```python
from build123d import *

# Parameters (mm, degrees)
F0_W        = 65.5969455838
F0_H        = 62.3628050089
F1_DEPTH    = 50.8
F3_DEPTH    = 101.6
F4_W        = 40.8792179078
F4_H        = 14.0294057783
F5_DEPTH    = 2.54
F6_R        = 5.8595306003
F7_DEPTH    = 25.4
F8_T1_DEPTH = 51.8777405358
F8_T3_DEPTH = 14.0294057783
F8_T5_DEPTH = 14.0294057783


# Not quite as in the source:
# - a fillet or chamfer that OpenCascade refuses, or shapes differently, is made with other operations: its cross-section is extruded or revolved along the edge and cut away or added


with BuildPart() as f1:
    # F0 (on Top) → F1 (new body)
    with BuildSketch(Plane.XY):
        with Locations((32.7984727919, 31.1814025044)):
            Rectangle(F0_W, F0_H)
    extrude(amount=F1_DEPTH)

    # F2 (on face) → F3 (cut)
    with BuildSketch(Plane.XZ):
        Polygon((89.7827520967, 45.4889908433), (33.5367023945, 62.9252642393), (74.5963230729, 21.5844195336), align=None)
    extrude(amount=-F3_DEPTH, mode=Mode.SUBTRACT)

    # F4 (on face) → F5 (cut)
    with BuildSketch(Plane(origin=(48.3447062482, 0, 48.0158379562), x_dir=(0, 1, 0), z_dir=(0.7095159293, 0, 0.7046893969))):
        with Locations((30.5939735845, -10.8757299604)):
            Rectangle(F4_W, F4_H)
    extrude(amount=-F5_DEPTH, mode=Mode.SUBTRACT)

    # F6 (on face) → F7 (cut)
    with BuildSketch(Plane.XZ):
        with Locations((31.5736755729, 25.0635799021)):
            Circle(F6_R)
    extrude(amount=-F7_DEPTH, mode=Mode.SUBTRACT)

    # F8: fillet of radius 5.08 on 4 edges, made by hand

    # F8_s2 → F8_t1 (join)
    with BuildSketch(Plane.XZ.offset(-62.0321051664)):
        with BuildLine():
            ThreePointArc((51.0655310864, 45.2763777457), (51.0565565883, 42.6467915619), (52.3635775369, 40.3650158763))
            Line((52.3635775369, 40.3650158763), (49.263360626, 43.4864666776))
            Line((49.263360626, 43.4864666776), (51.0655310864, 45.2763777457))
        make_face()
        with BuildLine():
            ThreePointArc((60.9519045829, 35.3222908675), (58.3223183991, 35.3312653655), (56.0495172115, 36.6538306007))
            Line((56.0495172115, 36.6538306007), (59.1497341225, 33.5323797994))
            Line((59.1497341225, 33.5323797994), (60.9519045829, 35.3222908675))
        make_face()
    extrude(amount=F8_T1_DEPTH)

    # F8_s4 → F8_t3 (join)
    with BuildSketch(Plane(origin=(12.6071983347, 0, -12.6935470887), x_dir=(0, 1, 0), z_dir=(-0.7046893969, 0, 0.7095159293))):
        with BuildLine():
            ThreePointArc((51.0335825384, -68.1375910703), (49.1741734871, -66.278182019), (46.6341734871, -65.5975910703))
            Line((46.6341734871, -65.5975910703), (51.0335825384, -65.5975910703))
            Line((51.0335825384, -65.5975910703), (51.0335825384, -68.1375910703))
        make_face()
    extrude(amount=F8_T3_DEPTH)

    # F8_s6 → F8_t5 (join)
    with BuildSketch(Plane(origin=(2.7208248382, 0, -2.7394602105), x_dir=(0, 1, 0), z_dir=(0.7046893969, 0, -0.7095159293))):
        with BuildLine():
            ThreePointArc((10.1543646306, 68.1375910703), (12.0137736818, 66.278182019), (14.5537736818, 65.5975910703))
            Line((14.5537736818, 65.5975910703), (10.1543646306, 65.5975910703))
            Line((10.1543646306, 65.5975910703), (10.1543646306, 68.1375910703))
        make_face()
    extrude(amount=F8_T5_DEPTH)


solid = f1.part
```
CAD build for the part. Positions are in the model's coordinates, mm. A direction names the side the tool comes from. Give positions to 0.01 mm unless a question says otherwise; leave off trailing zeros. Order: outer loops, then holes, each group sorted by start corner. A loop starts at its lowest first (then second) coordinate and runs counter-clockwise, first axis right, second up. Notation, with made-up numbers: M 24.5,56 L 79.5,56 A35 cw 79.5,89 Z; hole C 84.25,72.25 d5. An arc over 180 degrees is marked long. Put each result on its own line as item: value. Start each with the question number.
(1) Which spindle directions (+Z, -Z, +X, -X, +Y, -Y) get a long thin tool onto all of the face, cutting with end or side? Do faces 1 (the cylindrical face through (58.36, 30.88, 35.32)), 2 (the cylindrical face through (51.047, 30.88, 42.683)), 3 (the flat face through (32, 32, 0)). Say none if no direction does.
(2) Drill centre lines: line 1 along X through (y, z) = (5, 23); line 2 along Z through (x, y) = (46, 51); line 3 along Z through (x, y) = (48, 53). Where is each one in solid material? Low to high.
(3) Saw through at A-A, the plane z = 21.5. Write the cut outline in (x, y).
(4) Saw through at B-B, the plane y = 52.5. Write the cut outline in (x, z), then the cut area to 3 significant figures.
(5) Flat gauge pin, fed straight in: pin 1 Ø13 at (x, z) = (30, 27) entering from -Y. Where does the tip first touch, or does it go through?
(6) Saw through at D-D, the plane x = 46.5. Write the cut outline in (y, z), then the cut area to 3 significant figures.
(7) Saw through at C-C, the plane y = 4. Write the cut outline in (x, z), then the cut area to 3 significant figures.
(8) Mould opens along Y. For faces 4 (the flat face through (31, 25.4, 25)), 5 (the flat face through (54.181, 30.369, 38.535)), 6 (the cylindrical face through (54.87, 11.49, 39.3)), 7 (the cylindrical face through (36.986, 12.522, 22.819)) say: +Y half, -Y half, draft (parallel to the pull), parting line (faces both ways), or undercut.
Check result:
1. face 1: +Z
1. face 2: +X
1. face 3: -Z, +X, -X, +Y, -Y
2. line 1: x = 0 to 26.09, 37.06 to 65.6
2. line 2: z = 0 to 50.38
2. line 3: z = 0 to 48.36
3. outline: M 0,0 L 26.92,0 L 26.92,25.4 L 36.23,25.4 L 36.23,0 L 65.6,0 L 65.6,62.36 L 0,62.36 Z
4. outline: M 0,0 L 65.6,0 L 65.6,30.65 L 45.58,50.8 L 0,50.8 Z
4. area: 3,130 mm2
5. pin 1: stops at y = 0
6. outline: M 0,0 L 62.36,0 L 62.36,49.87 L 0,49.87 Z
6. area: 3,110 mm2
7. outline: M 0,0 L 65.6,0 L 65.6,30.65 L 45.58,50.8 L 0,50.8 Z; hole C 31.57,25.06 d11.72
7. area: 3,020 mm2
8. face 4: -Y half
8. face 5: undercut
8. face 6: undercut
8. face 7: draft
